```python
from build123d import *

# Parameters (mm, degrees)
BOSS_EXTRUDE1_DEPTH = 914.4
CUT_EXTRUDE2_REACH  = 14.7
SKETCH3_R           = 9.525
SKETCH3_R_2         = 10.31875
SKETCH3_R_3         = 11.1125
CUT_EXTRUDE3_REACH  = 14.7
SKETCH4_R           = 9.525
SKETCH5_R           = 11.1125
CUT_EXTRUDE4_DEPTH  = 102.6


with BuildPart() as part:
    # Sketch1 → Boss-Extrude1 (new body, symmetric)
    with BuildSketch(Plane.XY):
        with BuildLine():
            Line((0, 0), (0, 152.4))
            Line((0, 152.4), (0.00508, 152.4))
            ThreePointArc((0.00508, 152.4), (8.981744019, 148.681744019), (12.7, 139.70508))
            Line((12.7, 139.70508), (12.7, 25.4))
            ThreePointArc((12.7, 25.4), (16.419743879, 16.419743879), (25.4, 12.7))
            Line((25.4, 12.7), (88.90508, 12.7))
            ThreePointArc((88.90508, 12.7), (97.881744019, 8.981744019), (101.6, 0.00508))
            Line((101.6, 0.00508), (101.6, 0))
            Line((101.6, 0), (0, 0))
        make_face()
    extrude(amount=BOSS_EXTRUDE1_DEPTH, both=True)

    # Sketch3 → Cut-Extrude2 (cut, up to next)
    with BuildSketch(Plane(origin=(0, 12.7, 0), x_dir=(1, 0, 0), z_dir=(0, 1, 0)), mode=Mode.PRIVATE) as cut_extrude2_sk1:
        with Locations((63.5, -863.6)):
            Circle(SKETCH3_R)
    cut_extrude2_tool1 = extrude(cut_extrude2_sk1.sketch, amount=-CUT_EXTRUDE2_REACH, mode=Mode.PRIVATE) & part.part
    add(cut_extrude2_tool1.solids().sort_by_distance((63.5, 12.7, 863.6))[0], mode=Mode.SUBTRACT)
    # Sketch3 → Cut-Extrude2 (cut, up to next)
    with BuildSketch(Plane(origin=(0, 12.7, 0), x_dir=(1, 0, 0), z_dir=(0, 1, 0)), mode=Mode.PRIVATE) as cut_extrude2_sk2:
        with Locations((63.5, 863.6)):
            Circle(SKETCH3_R)
    cut_extrude2_tool2 = extrude(cut_extrude2_sk2.sketch, amount=-CUT_EXTRUDE2_REACH, mode=Mode.PRIVATE) & part.part
    add(cut_extrude2_tool2.solids().sort_by_distance((63.5, 12.7, -863.6))[0], mode=Mode.SUBTRACT)
    # Sketch3 → Cut-Extrude2 (cut, up to next)
    with BuildSketch(Plane(origin=(0, 12.7, 0), x_dir=(1, 0, 0), z_dir=(0, 1, 0)), mode=Mode.PRIVATE) as cut_extrude2_sk3:
        with Locations((63.5, -711.2)):
            Circle(SKETCH3_R_2)
    cut_extrude2_tool3 = extrude(cut_extrude2_sk3.sketch, amount=-CUT_EXTRUDE2_REACH, mode=Mode.PRIVATE) & part.part
    add(cut_extrude2_tool3.solids().sort_by_distance((63.5, 12.7, 711.2))[0], mode=Mode.SUBTRACT)
    # Sketch3 → Cut-Extrude2 (cut, up to next)
    with BuildSketch(Plane(origin=(0, 12.7, 0), x_dir=(1, 0, 0), z_dir=(0, 1, 0)), mode=Mode.PRIVATE) as cut_extrude2_sk4:
        with Locations((63.5, -457.2)):
            Circle(SKETCH3_R_2)
    cut_extrude2_tool4 = extrude(cut_extrude2_sk4.sketch, amount=-CUT_EXTRUDE2_REACH, mode=Mode.PRIVATE) & part.part
    add(cut_extrude2_tool4.solids().sort_by_distance((63.5, 12.7, 457.2))[0], mode=Mode.SUBTRACT)
    # Sketch3 → Cut-Extrude2 (cut, up to next)
    with BuildSketch(Plane(origin=(0, 12.7, 0), x_dir=(1, 0, 0), z_dir=(0, 1, 0)), mode=Mode.PRIVATE) as cut_extrude2_sk5:
        with Locations((63.5, -108.204)):
            Circle(SKETCH3_R_2)
    cut_extrude2_tool5 = extrude(cut_extrude2_sk5.sketch, amount=-CUT_EXTRUDE2_REACH, mode=Mode.PRIVATE) & part.part
    add(cut_extrude2_tool5.solids().sort_by_distance((63.5, 12.7, 108.204))[0], mode=Mode.SUBTRACT)
    # Sketch3 → Cut-Extrude2 (cut, up to next)
    with BuildSketch(Plane(origin=(0, 12.7, 0), x_dir=(1, 0, 0), z_dir=(0, 1, 0)), mode=Mode.PRIVATE) as cut_extrude2_sk6:
        with Locations((63.5, -533.4)):
            Circle(SKETCH3_R_2)
    cut_extrude2_tool6 = extrude(cut_extrude2_sk6.sketch, amount=-CUT_EXTRUDE2_REACH, mode=Mode.PRIVATE) & part.part
    add(cut_extrude2_tool6.solids().sort_by_distance((63.5, 12.7, 533.4))[0], mode=Mode.SUBTRACT)
    # Sketch3 → Cut-Extrude2 (cut, up to next)
    with BuildSketch(Plane(origin=(0, 12.7, 0), x_dir=(1, 0, 0), z_dir=(0, 1, 0)), mode=Mode.PRIVATE) as cut_extrude2_sk7:
        with Locations((63.5, -25.654)):
            Circle(SKETCH3_R_2)
    cut_extrude2_tool7 = extrude(cut_extrude2_sk7.sketch, amount=-CUT_EXTRUDE2_REACH, mode=Mode.PRIVATE) & part.part
    add(cut_extrude2_tool7.solids().sort_by_distance((63.5, 12.7, 25.654))[0], mode=Mode.SUBTRACT)
    # Sketch3 → Cut-Extrude2 (cut, up to next)
    with BuildSketch(Plane(origin=(0, 12.7, 0), x_dir=(1, 0, 0), z_dir=(0, 1, 0)), mode=Mode.PRIVATE) as cut_extrude2_sk8:
        with Locations((63.5, 228.346)):
            Circle(SKETCH3_R_3)
    cut_extrude2_tool8 = extrude(cut_extrude2_sk8.sketch, amount=-CUT_EXTRUDE2_REACH, mode=Mode.PRIVATE) & part.part
    add(cut_extrude2_tool8.solids().sort_by_distance((63.5, 12.7, -228.346))[0], mode=Mode.SUBTRACT)
    # Sketch3 → Cut-Extrude2 (cut, up to next)
    with BuildSketch(Plane(origin=(0, 12.7, 0), x_dir=(1, 0, 0), z_dir=(0, 1, 0)), mode=Mode.PRIVATE) as cut_extrude2_sk9:
        with Locations((63.5, -362.204)):
            Circle(SKETCH3_R_2)
    cut_extrude2_tool9 = extrude(cut_extrude2_sk9.sketch, amount=-CUT_EXTRUDE2_REACH, mode=Mode.PRIVATE) & part.part
    add(cut_extrude2_tool9.solids().sort_by_distance((63.5, 12.7, 362.204))[0], mode=Mode.SUBTRACT)
    # Sketch3 → Cut-Extrude2 (cut, up to next)
    with BuildSketch(Plane(origin=(0, 12.7, 0), x_dir=(1, 0, 0), z_dir=(0, 1, 0)), mode=Mode.PRIVATE) as cut_extrude2_sk10:
        with Locations((63.5, 812.8)):
            Circle(SKETCH3_R)
    cut_extrude2_tool10 = extrude(cut_extrude2_sk10.sketch, amount=-CUT_EXTRUDE2_REACH, mode=Mode.PRIVATE) & part.part
    add(cut_extrude2_tool10.solids().sort_by_distance((63.5, 12.7, -812.8))[0], mode=Mode.SUBTRACT)
    # Sketch3 → Cut-Extrude2 (cut, up to next)
    with BuildSketch(Plane(origin=(0, 12.7, 0), x_dir=(1, 0, 0), z_dir=(0, 1, 0)), mode=Mode.PRIVATE) as cut_extrude2_sk11:
        with Locations((63.5, -812.8)):
            Circle(SKETCH3_R)
    cut_extrude2_tool11 = extrude(cut_extrude2_sk11.sketch, amount=-CUT_EXTRUDE2_REACH, mode=Mode.PRIVATE) & part.part
    add(cut_extrude2_tool11.solids().sort_by_distance((63.5, 12.7, 812.8))[0], mode=Mode.SUBTRACT)

    # Sketch4 → Cut-Extrude3 (cut, up to next)
    with BuildSketch(Plane(origin=(12.7, 0, 0), x_dir=(0, 0, -1), z_dir=(1, 0, 0)), mode=Mode.PRIVATE) as cut_extrude3_sk1:
        with Locations((-850.9, 120.65)):
            Circle(SKETCH4_R)
    cut_extrude3_tool1 = extrude(cut_extrude3_sk1.sketch, amount=-CUT_EXTRUDE3_REACH, mode=Mode.PRIVATE) & part.part
    add(cut_extrude3_tool1.solids().sort_by_distance((12.7, 120.65, 850.9))[0], mode=Mode.SUBTRACT)
    # Sketch4 → Cut-Extrude3 (cut, up to next)
    with BuildSketch(Plane(origin=(12.7, 0, 0), x_dir=(0, 0, -1), z_dir=(1, 0, 0)), mode=Mode.PRIVATE) as cut_extrude3_sk2:
        with Locations((-596.9, 120.65)):
            Circle(SKETCH4_R)
    cut_extrude3_tool2 = extrude(cut_extrude3_sk2.sketch, amount=-CUT_EXTRUDE3_REACH, mode=Mode.PRIVATE) & part.part
    add(cut_extrude3_tool2.solids().sort_by_distance((12.7, 120.65, 596.9))[0], mode=Mode.SUBTRACT)
    # Sketch4 → Cut-Extrude3 (cut, up to next)
    with BuildSketch(Plane(origin=(12.7, 0, 0), x_dir=(0, 0, -1), z_dir=(1, 0, 0)), mode=Mode.PRIVATE) as cut_extrude3_sk3:
        with Locations((158.496, 127)):
            Circle(SKETCH4_R)
    cut_extrude3_tool3 = extrude(cut_extrude3_sk3.sketch, amount=-CUT_EXTRUDE3_REACH, mode=Mode.PRIVATE) & part.part
    add(cut_extrude3_tool3.solids().sort_by_distance((12.7, 127, -158.496))[0], mode=Mode.SUBTRACT)
    # Sketch4 → Cut-Extrude3 (cut, up to next)
    with BuildSketch(Plane(origin=(12.7, 0, 0), x_dir=(0, 0, -1), z_dir=(1, 0, 0)), mode=Mode.PRIVATE) as cut_extrude3_sk4:
        with Locations((762, 127)):
            Circle(SKETCH4_R)
    cut_extrude3_tool4 = extrude(cut_extrude3_sk4.sketch, amount=-CUT_EXTRUDE3_REACH, mode=Mode.PRIVATE) & part.part
    add(cut_extrude3_tool4.solids().sort_by_distance((12.7, 127, -762))[0], mode=Mode.SUBTRACT)

    # Sketch5 → Cut-Extrude4 (cut, through all)
    with BuildSketch(Plane.ZY):
        with Locations((-127, 38.1)):
            Circle(SKETCH5_R)
    extrude(amount=-CUT_EXTRUDE4_DEPTH, mode=Mode.SUBTRACT)


solid = part.part
```
Input: part model. Units: mm. Frame: model coordinates. A direction names the side the tool comes from. Coordinates: 2 decimals unless noted, no trailing zeros. Loops run counter-clockwise (first coordinate to the right, second up) from the corner with the lowest first, then second, coordinate; pieces in that order, holes last. Notation, with made-up numbers: M 55,48 L 71,48 A21 ccw 71,52 Z; hole C -33.75,-7 d3. An arc over 180 degrees is marked long. Use a Markdown table: item, result. Add a question column.
1) Pin query (flat end, axial travel): P1, Ø23.5, axis at x = 63.5, z = 108.204, coming from the -Y side; P2, Ø15, axis at x = 63.5, z = -863.6, coming from the +Y side; P3, Ø25, axis at x = 63.5, z = 863.6, coming from the +Y side; P4, Ø4, axis at y = 85, z = 116.5, coming from the +X side. Return the tip coordinate at first contact, or that it passes through.
2) Line query: L1, parallel to X at y = 66, z = 335.5; L2, parallel to Y at x = 4.5, z = -127. Output: solid intervals per line, ascending. Write a range as from..to.
3) Draft query along Z for faces 3 (the flat face through (10, 54, 914.4)), 4 (the flat face through (10, 54, -914.4)), 5 (the flat face through (52, 0, 13)). Return one class per face: +Z half, -Z half, draft (parallel to the pull), parting line (faces both ways), or undercut.
4) Set-up query: faces 1 (the flat face through (12.7, 83, 13)), 2 (the flat face through (0, 75, 13)). Return all of +Z, -Z, +X, -X, +Y, -Y with unobstructed straight access to the full face (end or side cutting, diameter ignored); none if empty.
5) Section B-B, the plane y = 69. Return the cut outline in (x, z).
Answer below:
| question | item | result |
|---|---|---|
| 1 | P1 | y = 0 |
| 1 | P2 | through |
| 1 | P3 | y = 12.7 |
| 1 | P4 | x = 12.7 |
| 2 | L1 | 0..12.7 |
| 2 | L2 | 0..26.99, 49.21..151.58 |
| 3 | face 3 | +Z half |
| 3 | face 4 | -Z half |
| 3 | face 5 | draft |
| 4 | face 1 | +Z, -Z, +X, +Y |
| 4 | face 2 | +Z, -Z, -X, +Y, -Y |
| 5 | outline | M 0,-914.4 L 12.7,-914.4 L 12.7,914.4 L 0,914.4 Z |
